Design review of the part built by this model. Coordinates are the model's own, in mm. Face numbers are marked on the shaded views. A direction names the side the tool comes from. Give positions to 0.01 mm unless a question says otherwise; leave off trailing zeros. Loops run counter-clockwise (first coordinate to the right, second up) from the corner with the lowest first, then second, coordinate; pieces in that order, holes last. Notation, with made-up numbers: (42.5, 33) -> (85.5, 33) arc R19 cw to (85.5, 37) -> close; hole circle Ø10 at (80, 15). An arc over 180 degrees is marked (long way). Answer as CSV lines item,"result".
from build123d import *

# Parameters (mm, degrees)
SKETCH1_W           = 990
SKETCH1_H           = 380
BOSS_EXTRUDE1_DEPTH = 12
SKETCH2_W           = 990
SKETCH2_H           = 25.4
BOSS_EXTRUDE2_DEPTH = 12.7
SKETCH3_W           = 990
SKETCH3_H           = 12
BOSS_EXTRUDE3_DEPTH = 60


with BuildPart() as part:
    # Sketch1 → Boss-Extrude1 (new body)
    with BuildSketch(Plane(origin=(0, 0, 0), x_dir=(1, 0, 0), z_dir=(0, 1, 0))):
        Rectangle(SKETCH1_W, SKETCH1_H)
    extrude(amount=BOSS_EXTRUDE1_DEPTH)

    # Sketch2 → Boss-Extrude2 (add)
    with BuildSketch(Plane.XZ):
        with Locations((0, 177.3)):
            Rectangle(SKETCH2_W, SKETCH2_H)
    extrude(amount=BOSS_EXTRUDE2_DEPTH)

    # Sketch3 → Boss-Extrude3 (add)
    with BuildSketch(Plane(origin=(0, 12, 0), x_dir=(1, 0, 0), z_dir=(0, 1, 0))):
        with Locations((0, 184)):
            Rectangle(SKETCH3_W, SKETCH3_H)
    extrude(amount=BOSS_EXTRUDE3_DEPTH)


solid = part.part
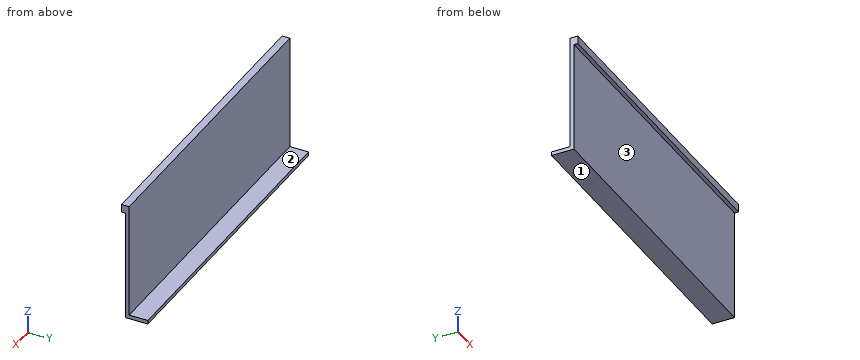
Q1. To check wall thickness, follow probe 1 along Z at (x, y) = (-372.5, 23); probe 2 along Y at (x, z) = (-97, 98.5); probe 3 along Z at (x, y) = (-407, -5.5). State the ranges of each line that lie inside material, in increasing order. Write a range as from..to.
Filled sheet:
probe 1,"z = -190..-178"
probe 2,"y = 0..12"
probe 3,"z = 164.6..190"
Q2. We need section A-A, the plane x = 421.5. State the section outline as (y, z) points.
Filled sheet:
outline,"(-12.7, 164.6) -> (0, 164.6) -> (0, -190) -> (72, -190) -> (72, -178) -> (12, -178) -> (12, 190) -> (-12.7, 190) -> close"
Q3. Clearance check with flat-ended pins moving along their axes: pin 1 Ø6.5 at (x, y) = (41.5, -9.5) entering from -Z; pin 2 Ø8 at (x, z) = (382, -31) entering from +Y; pin 3 Ø2 at (x, y) = (380.5, 23) entering from +Z. State where each tip first meets the part, or that it passes through.
Filled sheet:
pin 1,"stops at z = 164.6"
pin 2,"stops at y = 12"
pin 3,"stops at z = -178"
Q4. For the marked faces 1, 2 and 3, list the 3-axis set-ups (+Z, -Z, +X, -X, +Y, -Y) from which the entire face can be reached by the end or side of a thin tool; tool diameter is ignored.
Filled sheet:
face 1,"-Z, +X, -X, +Y, -Y"
face 2,"+Z, +X, -X, +Y"
face 3,"-Z, +X, -X, -Y"
Q5. We need section B-B, the plane z = -141.5. State the section outline as (x, y) points, and give its area (3 significant figures).
Filled sheet:
outline,"(-495, 0) -> (495, 0) -> (495, 12) -> (-495, 12) -> close"
area,"11,900 mm^2"
Q6. We need section C-C, the plane y = 60. State the section outline as (x, z) points.
Filled sheet:
outline,"(-495, -190) -> (495, -190) -> (495, -178) -> (-495, -178) -> close"
